from build123d import *

# Parameters (mm, degrees)
SKETCH1_W           = 60
SKETCH1_H           = 15
BOSS_EXTRUDE1_DEPTH = 20
SKETCH2_R           = 2.5
BOSS_EXTRUDE2_DEPTH = 12
SKETCH3_W           = 11
SKETCH3_H           = 16
BOSS_EXTRUDE3_DEPTH = 15
FILLET1_R           = 4
FILLET2_R           = 4
FILLET3_R           = 3


with BuildPart() as part:
    # Sketch1 → Boss-Extrude1 (new body)
    with BuildSketch(Plane(origin=(0, 0, 0), x_dir=(1, 0, 0), z_dir=(0, 1, 0))):
        Rectangle(SKETCH1_W, SKETCH1_H)
    extrude(amount=BOSS_EXTRUDE1_DEPTH)

    # Sketch2 → Boss-Extrude2 (add)
    with BuildSketch(Plane.XY.offset(7.5)):
        with Locations(Location((12, 10, 0), (0, 0, 180))):
            Circle(SKETCH2_R)
    extrude(amount=BOSS_EXTRUDE2_DEPTH)

    # Sketch3 → Boss-Extrude3 (add)
    with BuildSketch(Plane(origin=(30, 0, 0), x_dir=(0, 0, -1), z_dir=(1, 0, 0))):
        with Locations((0, 10)):
            Rectangle(SKETCH3_W, SKETCH3_H)
    extrude(amount=BOSS_EXTRUDE3_DEPTH)

    # Fillet1
    fillet1_edges = [part.edges().sort_by_distance(p)[0] for p in [
        (37.5, 18, 5.5),
        (37.5, 2, 5.5),
        (37.5, 2, -5.5),
        (37.5, 18, -5.5),
    ]]
    fillet(fillet1_edges, radius=FILLET1_R)

    # Fillet2
    fillet2_edges = [part.edges().sort_by_distance(p)[0] for p in [
        (45, 10, 5.5),
        (45, 18, 0),
        (45, 2, 0),
        (45, 10, -5.5),
        (45, 3.171572875, 4.328427125),
        (45, 3.171572875, -4.328427125),
        (45, 16.828427125, -4.328427125),
        (45, 16.828427125, 4.328427125),
    ]]
    fillet(fillet2_edges, radius=FILLET2_R)

    # Fillet3
    fillet3_edges = [part.edges().sort_by_distance(p)[0] for p in [
        (-30, 20, 0),
        (-30, 0, 0),
    ]]
    fillet(fillet3_edges, radius=FILLET3_R)


solid = part.part
The listing builds one solid part. Answer for the finished solid, in the listing's coordinates (mm). A direction names the side the tool comes from. Give positions to 0.01 mm unless a question says otherwise; leave off trailing zeros. Write each loop counter-clockwise with the first axis right and the second up, starting at its lowest first coordinate (ties: lowest second). Pieces come first, ordered by that corner, then holes. Notation, with made-up numbers: (-26.75, 38.5) - (4.25, 38.5) arc R30 ccw to (4.25, 68.5) - close; hole circle Ø1 at (-34, 72). An arc over 180 degrees is marked (long way). Use a Markdown table: item, result.
1. Section B-B on y = 10 is taken. Write down the section's boundary in (x, z), plus the area to 3 significant figures.
Values follow:
| item | result |
|---|---|
| outline | (-30, -7.5) - (30, -7.5) - (30, -5.5) - (41, -5.5) arc R4 ccw to (45, -1.5) - (45, 1.5) arc R4 ccw to (41, 5.5) - (30, 5.5) - (30, 7.5) - (14.5, 7.5) - (14.5, 19.5) - (9.5, 19.5) - (9.5, 7.5) - (-30, 7.5) - close |
| area | 1,120 mm² |
2. Section D-D on x = -6.5 is taken. Write down the section's boundary in (y, z).
Values follow:
| item | result |
|---|---|
| outline | (0, -7.5) - (20, -7.5) - (20, 7.5) - (0, 7.5) - close |
3. Section C-C on z = -3 is taken. Write down the section's boundary in (x, y), plus the area to 3 significant figures.
Values follow:
| item | result |
|---|---|
| outline | (-30, 3) arc R3 ccw to (-27, 0) - (30, 0) - (30, 2.29) - (41, 2.29) arc R3.71 ccw to (44.71, 6) - (44.71, 14) arc R3.71 ccw to (41, 17.71) - (30, 17.71) - (30, 20) - (-27, 20) arc R3 ccw to (-30, 17) - close |
| area | 1,420 mm² |
4. Section A-A on x = 12 is taken. Write down the section's boundary in (y, z).
Values follow:
| item | result |
|---|---|
| outline | (0, -7.5) - (20, -7.5) - (20, 7.5) - (12.5, 7.5) - (12.5, 19.5) - (7.5, 19.5) - (7.5, 7.5) - (0, 7.5) - close |
5. A tool of negligible diameter and unlimited length cuts with its end or side. For faces 1 (the cylindrical face through (35.577, 16.859, -4.297)), 2 (the flat face through (35, 10, -5.5)), 3 (the cylindrical face through (14, 11.5, 13.4)), 4 (the flat face through (30, 10, 7)), from which of +Z, -Z, +X, -X, +Y, -Y can it reach the whole face along a straight path? Write none if from no direction.
Values follow:
| item | result |
|---|---|
| face 1 | -Z, +X, +Y |
| face 2 | -Z, +X, +Y, -Y |
| face 3 | +Z |
| face 4 | +X |
6. Each of these flat-tipped pins is pushed along its axis until it touches: P1, Ø6.5, axis at x = 38, y = 11.5, coming from the +Z side; P2, Ø6.5, axis at x = 33.5, y = 11, coming from the -Z side; P3, Ø2.5, axis at x = 34, z = 0, coming from the -Y side. Where does it stop, or does it pass through?
Values follow:
| item | result |
|---|---|
| P1 | stops at z = 5.5 |
| P2 | stops at z = -5.5 |
| P3 | stops at y = 2 |
7. Find the intervals of material crossed by probe 1 along Z at (x, y) = (-3.5, 18); probe 2 along Z at (x, y) = (35, 12.75); probe 3 along X at (y, z) = (8.75, 7.25), in increasing order. Write a range as from..to.
Values follow:
| item | result |
|---|---|
| probe 1 | z = -7.5..7.5 |
| probe 2 | z = -5.5..5.5 |
| probe 3 | x = -30..30 |
